```python
from build123d import *

# Parameters (mm, degrees)
SKETCH1_R               = 1.5
BOSS_EXTRUDE1_DEPTH     = 95
CUT_EXTRUDE1_DEPTH      = 50
CUT_EXTRUDE1_DEPTH_BACK = 50
SKETCH3_R               = 0.8
FILLET1_R               = 0.5
SKETCH4_W               = 2.5
SKETCH4_H               = 3
CUT_EXTRUDE3_DEPTH      = 0.4


with BuildPart() as part:
    # Sketch1 → Boss-Extrude1 (new body)
    with BuildSketch(Plane.XY):
        with Locations((-5.911296371, 0)):
            Circle(SKETCH1_R)
    extrude(amount=BOSS_EXTRUDE1_DEPTH)

    # Sketch3 → Cut-Extrude1 (cut, two sides: drawn at the far end of the back side and taken through both)
    with BuildSketch(Plane(origin=(0, 0, 0), x_dir=(1, 0, 0), z_dir=(0, 1, 0)).offset(-CUT_EXTRUDE1_DEPTH_BACK)):
        with Locations(Location((-5.911296371, -1.5, 0), (0, 0, 90))):
            Circle(SKETCH3_R)
        with Locations(Location((-5.911296371, -93.5, 0), (0, 0, 90))):
            Circle(SKETCH3_R)
    extrude(amount=CUT_EXTRUDE1_DEPTH + CUT_EXTRUDE1_DEPTH_BACK, mode=Mode.SUBTRACT)

    # Fillet1
    fillet1_edges = [part.edges().sort_by_distance(p)[0] for p in [
        (-7.411296371, 0, 0),
        (-7.411296371, 0, 95),
    ]]
    fillet(fillet1_edges, radius=FILLET1_R)

    # Sketch4 → Cut-Extrude3 (cut)
    with BuildSketch(Plane(origin=(0, 1.5, 0), x_dir=(1, 0, 0), z_dir=(0, 1, 0))):
        with Locations((-5.911296371, -93.433012702)):
            Rectangle(SKETCH4_W, SKETCH4_H)
        with Locations((-5.911296371, -1.484191421)):
            Rectangle(SKETCH4_W, SKETCH4_H)
    extrude(amount=-CUT_EXTRUDE3_DEPTH, mode=Mode.SUBTRACT)


solid = part.part
```
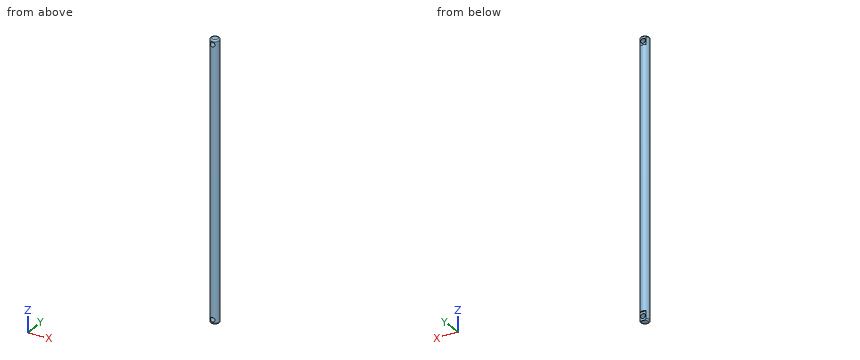
Build history of the part. All positions in model axes, mm. Coordinates: 2 decimals unless noted, no trailing zeros. Write each loop counter-clockwise with the first axis right and the second up, starting at its lowest first coordinate (ties: lowest second). Pieces come first, ordered by that corner, then holes.
1. Band-saw the part on B-B, the plane z = 63. Give the cut face in (x, y).
Answer block:
outline: circle Ø3 at (-5.91, 0)
2. Drill centre lines: probe 1 along Z at (x, y) = (-5.75, -0.3); probe 2 along X at (y, z) = (-0.1, 62.5); probe 3 along Z at (x, y) = (-5.15, 1.15). Where is each one in solid material? Low to high.
Answer block:
probe 1: z = 0 to 0.72, 2.28 to 92.72, 94.28 to 95
probe 2: x = -7.41 to -4.41
probe 3: z = 2.98 to 91.93
3. Drop a flat-ended pin along its axis: pin 1 (1 mm diameter, centred on x = -6, z = 2, fed in from +Y). Give the stop position or say it passes through.
Answer block:
pin 1: stops at y = 1.1
4. Band-saw the part on A-A, the plane z = 1.5. Give the cut face in (x, y).
Answer block:
outline: (-6.93, 1.1) arc R1.5 ccw to (-6.71, -1.27) - (-6.71, 1.1) - close; (-5.11, -1.27) arc R1.5 ccw to (-4.89, 1.1) - (-5.11, 1.1) - close
